Job drawing, mm, ordinate dimensions from the low corner. One solid piece. A direction names the side the tool comes from. Give positions to 0.01 mm unless a question says otherwise; leave off trailing zeros. Write each loop counter-clockwise with the first axis right and the second up, starting at its lowest first coordinate (ties: lowest second). Pieces come first, ordered by that corner, then holes. Notation, with made-up numbers: M 71.25,63.25 L 79.25,63.25 A12 ccw 79.25,79.25 Z; hole C -35.5,-7.75 d8. An arc over 180 degrees is marked long. Answer as CSV lines item,"result". Start each with the question number.
Item 1: Pin check, flat tips, straight feed: pin 1 (1.6 mm diameter, centred on x = 0.5, y = 1, fed in from +Z) (1 decimal); pin 2 (0.8 mm diameter, centred on x = 1, y = 9.5, fed in from +Z) (3 decimals); pin 3 (1.6 mm diameter, centred on x = 0.5, y = 9.5, fed in from -Z) (3 decimals). Stop position of each tip, or through.
Item 2: 3-axis set-ups, long thin cutter, end or side, ignore diameter. For the marked faces 1, 2, 3 and 4: which of +Z, -Z, +X, -X, +Y, -Y reach the whole face in a straight line?
Item 3: Wall check: L1, parallel to X at y = 8.75, z = 4; L2, parallel to Y at x = 4, z = 3.75; L3, parallel to Z at x = 0.6, y = 9.5 (1 decimal). Give the ranges that are in metal, low to high. Write a range as from..to.
Item 4: Band-saw the part on B-B, the plane y = 9.25. List the corners of the cut face in (x, z) (1 decimal).
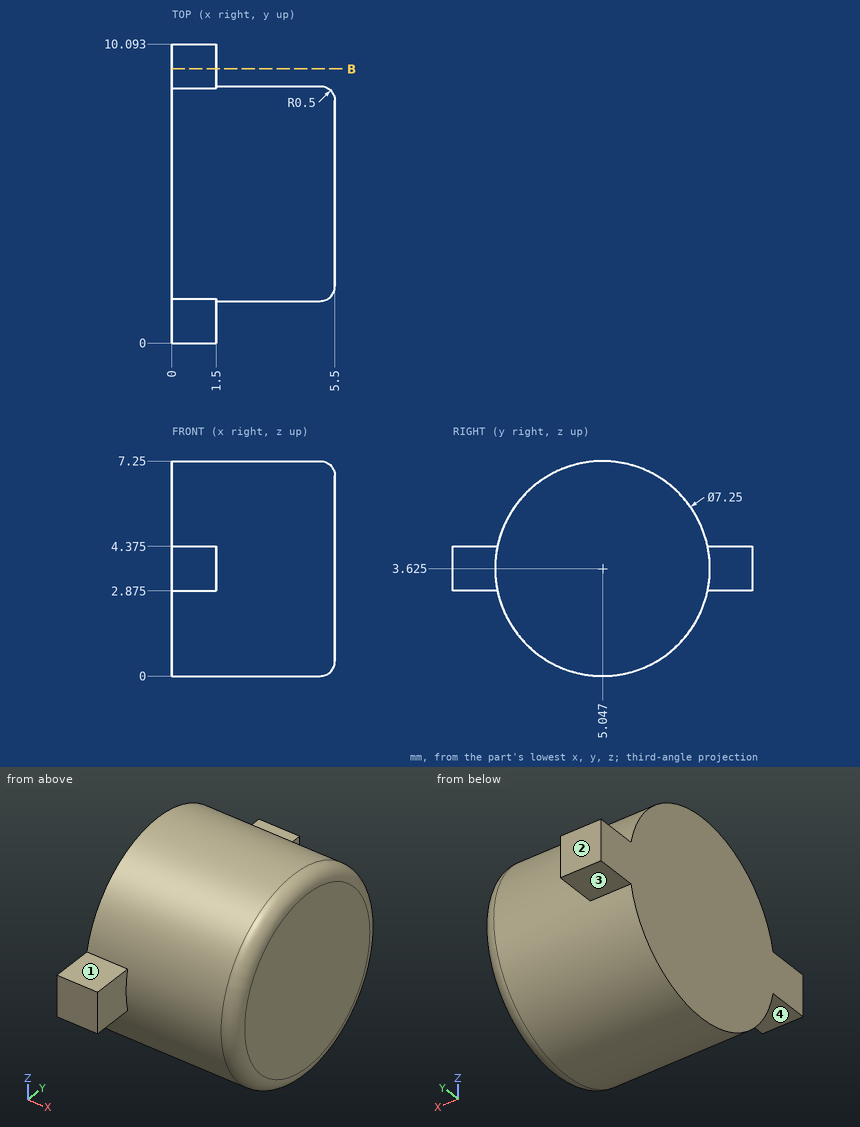
Output:
1,pin 1,"z = 5.2"
1,pin 2,"z = 4.375"
1,pin 3,"z = 2.875"
2,face 1,"+Z, +X, -X, -Y"
2,face 2,"+Z, -Z, +X, -X, +Y"
2,face 3,"-Z, +X, -X, +Y"
2,face 4,"-Z, +X, -X, -Y"
3,L1,"0..1.5"
3,L2,"1.42..8.67"
3,L3,"2.9..4.4"
4,outline,"M 0,2.9 L 1.5,2.9 L 1.5,4.4 L 0,4.4 Z"
